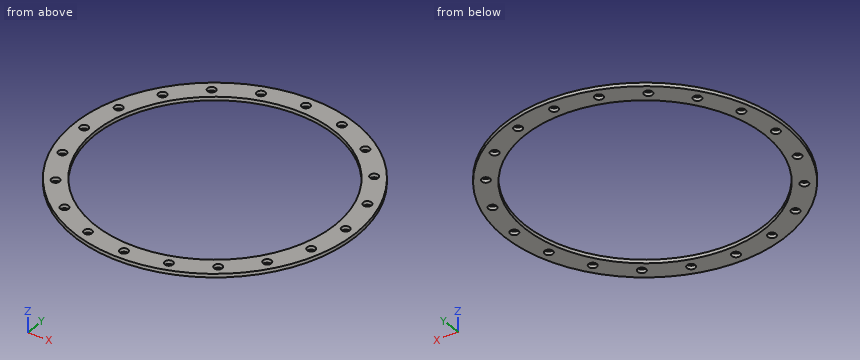
from build123d import *

# Parameters (mm, degrees)
F0_R     = 380.9121654934
F0_R_2   = 324.6612464713
F2_DEPTH = 9.525
F5_D     = 22.225


# Not quite as in the source:
# - a feature names something its author has since deleted; it is built from what else it names
# - the program builds the solid bodies; features that only make, move or delete a surface that nothing else refers to are left out


with BuildPart() as f2:
    # F0 (on Top) → F2 (new body)
    with BuildSketch(Plane.XY):
        Circle(F0_R)
        Circle(F0_R_2, mode=Mode.SUBTRACT)
    extrude(amount=F2_DEPTH)

    # F5 (through all)
    with Locations(Plane(origin=(0, 0, 0), x_dir=(1, 0, 0), z_dir=(0, 0, -1))):
        with Locations((-285.2887655833, -207.2744209584), (-335.3770581092, -108.9706118443), (-352.636307478, 0), (-335.3770581092, 108.9706118443), (-285.2887655833, 207.2744209584), (-207.2744209584, 285.2887655833), (-108.9706118443, 335.3770581092), (0, 352.636307478), (108.9706118443, 335.3770581092), (207.2744209584, 285.2887655833), (285.2887655833, 207.2744209584), (335.3770581092, 108.9706118443), (352.636307478, 0), (335.3770581092, -108.9706118443), (285.2887655833, -207.2744209584), (207.2744209584, -285.2887655833), (108.9706118443, -335.3770581092), (0, -352.636307478), (-108.9706118443, -335.3770581092), (-207.2744209584, -285.2887655833)):
            Hole(F5_D / 2)


solid = f2.part
Model file for the job. Use its own axes, mm. Give positions to 0.01 mm unless a question says otherwise; leave off trailing zeros. Loops run counter-clockwise (first coordinate to the right, second up) from the corner with the lowest first, then second, coordinate; pieces in that order, holes last.
Item 1: Slice it at C-C (x = -314). Write the cut outline in (y, z) (3 decimals).
Check values:
outline: (-215.634, 0) - (-82.516, 0) - (-82.516, 9.525) - (-215.634, 9.525) - close; (82.516, 0) - (215.634, 0) - (215.634, 9.525) - (82.516, 9.525) - close
Item 2: Slice it at A-A (y = 0). Write the cut outline in (x, z) (3 decimals).
Check values:
outline: (-380.912, 0) - (-363.749, 0) - (-363.749, 9.525) - (-380.912, 9.525) - close; (-341.524, 0) - (-324.661, 0) - (-324.661, 9.525) - (-341.524, 9.525) - close; (324.661, 0) - (341.524, 0) - (341.524, 9.525) - (324.661, 9.525) - close; (363.749, 0) - (380.912, 0) - (380.912, 9.525) - (363.749, 9.525) - close
Item 3: Drill centre lines: line 1 along X through (y, z) = (-108, 8.75); line 2 along X through (y, z) = (294, 2) (3 decimals); line 3 along Y through (x, z) = (109, 4.75). Where is each one in solid material? Low to high.
Check values:
line 1: x = -365.28 to -346.45, -324.31 to -306.17, 306.17 to 324.31, 346.45 to 365.28
line 2: x = -242.194 to -214.174, -200.375 to -137.728, 137.728 to 200.375, 214.174 to 242.194
line 3: y = -364.98 to -346.49, -324.26 to -305.82, 305.82 to 324.26, 346.49 to 364.98
Item 4: Slice it at D-D (z = 6.25). Give the number of separate pieces and of enclosed holes in the cut face, plus the area to 3 significant figures.
Check values:
separate pieces: 1
enclosed holes: 21
area: 117,000 mm2
Item 5: Drop flat-ended pins along their axis: P1, Ø18, axis at x = 285.29, y = 207.27, coming from the -Z side; P2, Ø4, axis at x = 124, z = 4.5, coming from the +Y side; P3, Ø2, axis at y = -37, z = 1.5, coming from the -X side; P4, Ø3, axis at y = 130.5, z = 2, coming from the +X side. Give the stop position or say it passes through.
Check values:
P1: passes through
P2: stops at y = 360.85
P3: stops at x = -379.21
P4: stops at x = 358.4
